Build history of the part. All positions in model axes, mm. A direction names the side the tool comes from. Round coordinates to 2 decimals unless told otherwise and drop trailing zeros. Write each loop counter-clockwise with the first axis right and the second up, starting at its lowest first coordinate (ties: lowest second). Pieces come first, ordered by that corner, then holes. Notation, with made-up numbers: (-13.75, 77) - (11.25, 77) arc R17 cw to (11.25, 99) - close; hole circle Ø8 at (56, 26.25). An arc over 180 degrees is marked (long way). Write each question's results on one line, items separated by ' | '.
Autodesk Inventor part; units mm, degrees
ref_plane "YZ Plane" through (0, 0, 0) normal (1, 0, 0) x (0, 1, 0)
ref_plane "XZ Plane" through (0, 0, 0) normal (0, 1, 0) x (-1, 0, 0)
ref_plane "XY Plane" through (0, 0, 0) normal (0, 0, 1) x (1, 0, 0)
sketch "Sketch1" plane through (0, 0, 0) normal (0, 0, 1) x (1, 0, 0)
  line L0 (0, 0) -> (457.2, 0)
  line L1 (457.2, 0) -> (457.2, 139.7)
  line L2 (457.2, 139.7) -> (0, 139.7)
  line L3 (0, 139.7) -> (0, 0)
  dimension "d0" = 457.2
  dimension "d1" = 139.7
extrude "Extrusion1" add sketch "Sketch1" along normal blind 3.175
sketch "Sketch2" plane through (0, 0, 3.175) normal (0, 0, 1) x (1, 0, 0)
  line L0 (0, 139.7) -> (0, 0)
  line L1 (0, 114.3) -> (457.2, 114.3)
  line L2 (457.2, 139.7) -> (0, 139.7)
  line L3 (0, 38.1) -> (457.2, 38.1)
  line L4 (457.2, 0) -> (457.2, 139.7)
  line L5 (0, 0) -> (457.2, 0)
  line L6 (12.7, 17.6917) -> (50.8, 17.6917)
  line L7 (50.8, 17.6917) -> (50.8, 14.5167)
  line L8 (50.8, 14.5167) -> (12.7, 14.5167)
  line L9 (12.7, 14.5167) -> (12.7, 17.6917)
  line L10 (12.7, 127) -> (50.8, 127)
  line L11 (50.8, 127) -> (50.8, 123.825)
  line L12 (50.8, 123.825) -> (12.7, 123.825)
  line L13 (12.7, 123.825) -> (12.7, 127)
  line L14 (76.2, 127) -> (114.3, 127)
  line L15 (114.3, 127) -> (114.3, 123.825)
  line L16 (114.3, 123.825) -> (76.2, 123.825)
  line L17 (76.2, 123.825) -> (76.2, 127)
  line L18 (139.7, 127) -> (177.8, 127)
  line L19 (177.8, 127) -> (177.8, 123.825)
  line L20 (177.8, 123.825) -> (139.7, 123.825)
  line L21 (139.7, 123.825) -> (139.7, 127)
  line L22 (203.2, 127) -> (241.3, 127)
  line L23 (241.3, 127) -> (241.3, 123.825)
  line L24 (241.3, 123.825) -> (203.2, 123.825)
  line L25 (203.2, 123.825) -> (203.2, 127)
  line L26 (266.7, 127) -> (304.8, 127)
  line L27 (304.8, 127) -> (304.8, 123.825)
  line L28 (304.8, 123.825) -> (266.7, 123.825)
  line L29 (266.7, 123.825) -> (266.7, 127)
  line L30 (330.2, 127) -> (368.3, 127)
  line L31 (368.3, 127) -> (368.3, 123.825)
  line L32 (368.3, 123.825) -> (330.2, 123.825)
  line L33 (330.2, 123.825) -> (330.2, 127)
  line L34 (393.7, 127) -> (431.8, 127)
  line L35 (431.8, 127) -> (431.8, 123.825)
  line L36 (431.8, 123.825) -> (393.7, 123.825)
  line L37 (393.7, 123.825) -> (393.7, 127)
  line L38 (76.2, 17.6917) -> (114.3, 17.6917)
  line L39 (114.3, 17.6917) -> (114.3, 14.5167)
  line L40 (114.3, 14.5167) -> (76.2, 14.5167)
  line L41 (76.2, 14.5167) -> (76.2, 17.6917)
  line L42 (139.7, 17.6917) -> (177.8, 17.6917)
  line L43 (177.8, 17.6917) -> (177.8, 14.5167)
  line L44 (177.8, 14.5167) -> (139.7, 14.5167)
  line L45 (139.7, 14.5167) -> (139.7, 17.6917)
  line L46 (203.2, 17.6917) -> (241.3, 17.6917)
  line L47 (241.3, 17.6917) -> (241.3, 14.5167)
  line L48 (241.3, 14.5167) -> (203.2, 14.5167)
  line L49 (203.2, 14.5167) -> (203.2, 17.6917)
  line L50 (266.7, 17.6917) -> (304.8, 17.6917)
  line L51 (304.8, 17.6917) -> (304.8, 14.5167)
  line L52 (304.8, 14.5167) -> (266.7, 14.5167)
  line L53 (266.7, 14.5167) -> (266.7, 17.6917)
  line L54 (330.2, 17.6917) -> (368.3, 17.6917)
  line L55 (368.3, 17.6917) -> (368.3, 14.5167)
  line L56 (368.3, 14.5167) -> (330.2, 14.5167)
  line L57 (330.2, 14.5167) -> (330.2, 17.6917)
  line L58 (393.7, 17.6917) -> (431.8, 17.6917)
  line L59 (431.8, 17.6917) -> (431.8, 14.5167)
  line L60 (431.8, 14.5167) -> (393.7, 14.5167)
  line L61 (393.7, 14.5167) -> (393.7, 17.6917)
  dimension "d106" = 3.175
  dimension "d107" = 25.4
  dimension "d108" = 25.4
  dimension "d109" = 12.7
  dimension "d110" = 12.7
  dimension "d111" = 25.4
  dimension "d112" = 12.7
  dimension "d113" = 25.4
  dimension "d114" = 12.7
  dimension "d115" = 25.4
  dimension "d116" = 12.7
  dimension "d117" = 25.4
  dimension "d118" = 12.7
  dimension "d119" = 25.4
  dimension "d120" = 12.7
  dimension "d121" = 12.7
  dimension "d122" = 38.1
  dimension "d123" = 38.1
  dimension "d124" = 38.1
  dimension "d125" = 38.1
  dimension "d126" = 38.1
  dimension "d127" = 38.1
  dimension "d128" = 3.175
  dimension "d129" = 3.175
  dimension "d130" = 3.175
  dimension "d131" = 3.175
  dimension "d132" = 3.175
  dimension "d133" = 3.175
  dimension "d134" = 25.4
  dimension "d135" = 38.1
  dimension "d136" = 25.4
  dimension "d137" = 38.1
  dimension "d138" = 25.4
  dimension "d139" = 38.1
  dimension "d140" = 25.4
  dimension "d141" = 38.1
  dimension "d142" = 25.4
  dimension "d143" = 38.1
  dimension "d144" = 25.4
  dimension "d145" = 38.1
  dimension "d146" = 25.4
  dimension "d147" = 38.1
  dimension "d148" = 14.5167
  dimension "d150" = 14.5167
  dimension "d151" = 3.175
  dimension "d152" = 3.175
extrude "Extrusion2" cut sketch "Sketch2" against normal through all contours L6 L7 L8 L9 | L10 L11 L12 L13 | L14 L15 L16 L17 | L18 L19 L20 L21 | L22 L23 L24 L25 | L26 L27 L28 L29 | L30 L31 L32 L33 | L34 L35 L36 L37 | L38 L39 L40 L41 | L42 L43 L44 L45 | L46 L47 L48 L49 | L50 L51 L52 L53 | L54 L55 L56 L57 | L58 L59 L60 L61
sketch "Sketch3" plane through (0, 0, 3.175) normal (0, 0, 1) x (1, 0, 0)
  line L0 (0, 139.7) -> (0, 0)
  line L1 (0, 38.1) -> (457.2, 38.1)
  line L2 (457.2, 0) -> (457.2, 139.7)
  line L3 (0, 0) -> (457.2, 0)
  line L4 (0, 101.6) -> (457.2, 101.6)
  line L5 (457.2, 139.7) -> (0, 139.7)
  line L6 (12.7, 88.9) -> (12.7, 38.1)
  line L7 (12.7, 38.1) -> (63.5, 38.1)
  line L8 (63.5, 38.1) -> (12.7, 88.9)
  line L9 (29.5512, 90.0093) -> (80.3512, 39.2093)
  line L10 (80.3512, 39.2093) -> (80.3512, 90.0093)
  line L11 (80.3512, 90.0093) -> (29.5512, 90.0093)
  line L12 (93.0512, 38.1) -> (93.0512, 88.9)
  line L13 (93.0512, 38.1) -> (143.8512, 38.1)
  line L14 (143.8512, 38.1) -> (93.0512, 88.9)
  line L15 (111.0117, 88.9) -> (161.8117, 88.9)
  line L16 (161.8117, 88.9) -> (161.8117, 38.1)
  line L17 (161.8117, 38.1) -> (111.0117, 88.9)
  line L18 (174.5117, 88.9) -> (174.5117, 38.1)
  line L19 (174.5117, 38.1) -> (225.3117, 38.1)
  line L20 (225.3117, 38.1) -> (174.5117, 88.9)
  line L21 (243.2722, 38.1) -> (243.2722, 88.9)
  line L22 (243.2722, 88.9) -> (192.4722, 88.9)
  line L23 (192.4722, 88.9) -> (243.2722, 38.1)
  line L24 (255.9722, 88.9) -> (255.9722, 38.1)
  line L25 (255.9722, 38.1) -> (306.7722, 38.1)
  line L26 (306.7722, 38.1) -> (255.9722, 88.9)
  line L27 (273.9327, 88.9) -> (324.7327, 88.9)
  line L28 (324.7327, 88.9) -> (324.7327, 38.1)
  line L29 (324.7327, 38.1) -> (273.9327, 88.9)
  line L30 (337.4327, 88.9) -> (337.4327, 38.1)
  line L31 (337.4327, 38.1) -> (388.2327, 38.1)
  line L32 (388.2327, 38.1) -> (337.4327, 88.9)
  line L33 (355.3933, 88.9) -> (406.1933, 88.9)
  line L34 (406.1933, 88.9) -> (406.1933, 38.1)
  line L35 (406.1933, 38.1) -> (355.3933, 88.9)
  line L36 (425.2433, 88.9) -> (437.9433, 88.9)
  line L37 (437.9433, 88.9) -> (437.9433, 38.1)
  line L38 (437.9433, 38.1) -> (425.2433, 38.1)
  line L39 (425.2433, 38.1) -> (425.2433, 88.9)
  point P0 (355.3933, 88.9)
  dimension "d43" = 38.1
  dimension "d44" = 38.1
  dimension "d47" = 12.7
  dimension "d49" = 50.8
  dimension "d52" = 12.7
  dimension "d55" = 50.8
  dimension "d62" = 50.8
  dimension "d64" = 12.7
  dimension "d65" = 12.7
  dimension "d66" = 50.8
  dimension "d67" = 50.8
  dimension "d68" = 12.7
  dimension "d69" = 12.7
  dimension "d71" = 50.8
  dimension "d72" = 50.8
  dimension "d73" = 12.7
  dimension "d74" = 12.7
  dimension "d75" = 50.8
  dimension "d76" = 12.7
  dimension "d77" = 12.7
  dimension "d78" = 50.8
  dimension "d79" = 50.8
  dimension "d80" = 12.7
  dimension "d81" = 12.7
  dimension "d82" = 50.8
  dimension "d83" = 50.8
  dimension "d84" = 12.7
  dimension "d85" = 12.7
  dimension "d86" = 50.8
  dimension "d87" = 50.8
  dimension "d89" = 12.7
  dimension "d90" = 12.7
  dimension "d91" = 12.7
  dimension "d92" = 50.8
  dimension "d93" = 50.8
  dimension "d94" = 50.8
  dimension "d96" = 19.05
  dimension "d153" = 0
  dimension "d154" = 0
extrude "Extrusion3" cut sketch "Sketch3" against normal through all contours L17 L15 L16 | L23 L22 L21 | L29 L27 L28 | L35 L33 L34 | L6 L8 L1 | L1 L39 L36 L37 | L12 L14 L1 | L1 L30 L32 | L18 L20 L1 | L1 L24 L26 | L11 L10 L9
properties part number "Bridge2"
(1) Drill centre lines: probe 1 along Y at (x, z) = (333, 2.45) (3 decimals); probe 2 along Y at (x, z) = (435.5, 1.8); probe 3 along Y at (x, z) = (339, 2.45) (3 decimals). Where is each one in solid material? Low to high. Write a range as [from, to].
Worked answers:
probe 1: y = [0, 14.517], [17.692, 123.825], [127, 139.7] | probe 2: y = [0, 38.1], [88.9, 139.7] | probe 3: y = [0, 14.517], [17.692, 38.1], [87.333, 123.825], [127, 139.7]
(2) Two-plate mould, pull along Y, no slides. Class faces 3 (the flat face through (225, 55, 0)), 4 (the flat face through (217.517, 63.856, 1.61)): released by +Y, released by -Y, zero draft, split by the parting line, or undercut.
Worked answers:
face 3: zero draft | face 4: undercut
(3) Slice it at C-C, the plane z = 1.7. State how many separate pieces and enclosed holes the cut face has, and give its area (3 significant figures).
Worked answers:
separate pieces: 1 | enclosed holes: 25 | area: 48,600 mm2
(4) Tool access for faces 1 (the flat face through (225, 55, 3.175)), 2 (the flat face through (54.6, 64.96, 1.61)): list every direction of +Z, -Z, +X, -X, +Y, -Y with a clear straight run to the whole face (end or side of a thin tool).
Worked answers:
face 1: +Z, +X, -X, +Y, -Y | face 2: +Z, -Z
(5) Slice it at A-A, the plane x = 211. Write the cut outline in (y, z) (3 decimals).
Worked answers:
outline: (0, 0) - (14.517, 0) - (14.517, 3.175) - (0, 3.175) - close; (17.692, 0) - (38.1, 0) - (38.1, 3.175) - (17.692, 3.175) - close; (52.412, 0) - (70.372, 0) - (70.372, 3.175) - (52.412, 3.175) - close; (88.9, 0) - (123.825, 0) - (123.825, 3.175) - (88.9, 3.175) - close; (127, 0) - (139.7, 0) - (139.7, 3.175) - (127, 3.175) - close
(6) Slice it at B-B, the plane x = 376.5. Write the cut outline in (y, z) (3 decimals).
Worked answers:
outline: (0, 0) - (38.1, 0) - (38.1, 3.175) - (0, 3.175) - close; (49.833, 0) - (67.793, 0) - (67.793, 3.175) - (49.833, 3.175) - close; (88.9, 0) - (139.7, 0) - (139.7, 3.175) - (88.9, 3.175) - close
